Geometry: final body of the model. Coordinates: model frame, mm. A direction names the side the tool comes from. Coordinates: 2 decimals unless noted, no trailing zeros. Order: outer loops, then holes, each group sorted by start corner. A loop starts at its lowest first (then second) coordinate and runs counter-clockwise, first axis right, second up. Notation, with made-up numbers: M 61.25,3.5 L 71.25,3.5 A18 cw 71.25,23.5 Z; hole C -31,-20.75 d6. An arc over 180 degrees is marked long. Write item = value, one per line.
from build123d import *

# Parameters (mm, degrees)
ESBO_O1_R                  = 8
RESSALTO_EXTRUS_O1_DEPTH   = 15
CORTE_EXTRUS_O1_DEPTH      = 26.82634314
CORTE_EXTRUS_O1_DEPTH_BACK = 26.82634314
ESBO_O2_R                  = 1.5


with BuildPart() as part:
    # Esboço1 → Ressalto-extrusão1 (new body)
    with BuildSketch(Plane.XY):
        with BuildLine():
            Line((2, 12.866068747), (-2, 12.866068747))
            Line((-2, 12.866068747), (-2, 14.866068747))
            ThreePointArc((-2, 14.866068747), (-10.606601718, 10.606601718), (-14.866068747, 2))
            Line((-14.866068747, 2), (-12.866068747, 2))
            Line((-12.866068747, 2), (-12.866068747, -2))
            Line((-12.866068747, -2), (-14.866068747, -2))
            ThreePointArc((-14.866068747, -2), (-10.606601718, -10.606601718), (-2, -14.866068747))
            Line((-2, -14.866068747), (-2, -12.866068747))
            Line((-2, -12.866068747), (2, -12.866068747))
            Line((2, -12.866068747), (2, -14.866068747))
            ThreePointArc((2, -14.866068747), (10.606601718, -10.606601718), (14.866068747, -2))
            Line((14.866068747, -2), (12.866068747, -2))
            Line((12.866068747, -2), (12.866068747, 2))
            Line((12.866068747, 2), (14.866068747, 2))
            ThreePointArc((14.866068747, 2), (10.606601718, 10.606601718), (2, 14.866068747))
            Line((2, 14.866068747), (2, 12.866068747))
        make_face()
        Circle(ESBO_O1_R, mode=Mode.SUBTRACT)
    extrude(amount=RESSALTO_EXTRUS_O1_DEPTH)

    # Esboço2 → Corte-extrusão1 (cut, two sides: drawn at the far end of the back side and taken through both)
    with BuildSketch(Plane(origin=(0, 0, 0), x_dir=(0, 0, -1), z_dir=(1, 0, 0)).offset(-CORTE_EXTRUS_O1_DEPTH_BACK)):
        with Locations((-9, 0)):
            Circle(ESBO_O2_R)
    extrude(amount=CORTE_EXTRUS_O1_DEPTH + CORTE_EXTRUS_O1_DEPTH_BACK, mode=Mode.SUBTRACT)


solid = part.part
1) Pin query (flat end, axial travel): pin 1 (2 mm diameter, centred on x = -7, z = 7, fed in from -Y); pin 2 (0.6 mm diameter, centred on y = -13.5, z = 9, fed in from -X); pin 3 (2 mm diameter, centred on y = -14, z = 6.5, fed in from +X). Return the tip coordinate at first contact, or that it passes through.
Numbers:
pin_1 = -13.75
pin_2 = -7.12
pin_3 = 7.48
2) Section D-D, the plane z = 12.25. Return loops of the section in (x, y), and give its area (3 significant figures).
Numbers:
outline = M -14.87,-2 A15 ccw -2,-14.87 L -2,-12.87 L 2,-12.87 L 2,-14.87 A15 ccw 14.87,-2 L 12.87,-2 L 12.87,2 L 14.87,2 A15 ccw 2,14.87 L 2,12.87 L -2,12.87 L -2,14.87 A15 ccw -14.87,2 L -12.87,2 L -12.87,-2 Z; hole C 0,0 d16
area = 472 mm²
3) Section B-B, the plane x = 0. Return loops of the section in (y, z), and give its area (3 significant figures).
Numbers:
outline = M -12.87,0 L -8,0 L -8,15 L -12.87,15 Z; M 8,0 L 12.87,0 L 12.87,15 L 8,15 Z
area = 146 mm²
4) Line query: L1, parallel to Y at x = 0, z = 6; L2, parallel to Z at x = 10.7, y = 0. Output: solid intervals per line, ascending.
Numbers:
L1 = -12.87 to -8, 8 to 12.87
L2 = 0 to 7.5, 10.5 to 15
5) Mould query, pull axis Y, two halves, no side actions, for faces 4 (the face through (-14, -2, 7)), 5 (the face through (10.51, -10.7, 7.4)), 6 (the face through (10.7, 10.51, 7.4)). Classes: pulls with the +Y half, pulls with the -Y half, needs draft (parallel to the pull), parting line crosses it, or undercut.
Numbers:
face_4 = undercut
face_5 = pulls with the -Y half
face_6 = pulls with the +Y half
6) Section C-C, the plane z = 9. Return loops of the section in (x, y).
Numbers:
outline = M -14.87,-2 A15 ccw -2,-14.87 L -2,-12.87 L 2,-12.87 L 2,-14.87 A15 ccw 14.87,-2 L 12.87,-2 L 12.87,-1.5 L 7.86,-1.5 A8 cw -7.86,-1.5 L -12.87,-1.5 L -12.87,-2 Z; M -14.87,2 L -12.87,2 L -12.87,1.5 L -7.86,1.5 A8 cw 7.86,1.5 L 12.87,1.5 L 12.87,2 L 14.87,2 A15 ccw 2,14.87 L 2,12.87 L -2,12.87 L -2,14.87 A15 ccw Z
7) Section A-A, the plane y = 0. Return loops of the section in (x, z).
Numbers:
outline = M -12.87,0 L -8,0 L -8,7.5 L -12.87,7.5 Z; M -12.87,10.5 L -8,10.5 L -8,15 L -12.87,15 Z; M 8,0 L 12.87,0 L 12.87,7.5 L 8,7.5 Z; M 8,10.5 L 12.87,10.5 L 12.87,15 L 8,15 Z
8) Set-up query: faces 1 (the face through (0, 12.866, 7)), 2 (the face through (14, -2, 7)), 3 (the face through (-2, -14, 7)). Return all of +Z, -Z, +X, -X, +Y, -Y with unobstructed straight access to the full face (end or side cutting, diameter ignored); none if empty.
Numbers:
face_1 = +Z, -Z, +Y
face_2 = +Z, -Z, +X
face_3 = +Z, -Z, -Y
